Here's how the part is built. I have some questions about the finished solid (model axes, mm). Coordinates: 2 decimals unless noted, no trailing zeros. Order: outer loops, then holes, each group sorted by start corner. A loop starts at its lowest first (then second) coordinate and runs counter-clockwise, first axis right, second up.
```python
from build123d import *

# Parameters (mm, degrees)
SKETCH_1_R      = 12.5
SKETCH_1_R_2    = 4
SKETCH_1_R_3    = 1.5
SKETCH_1_R_4    = 1
SKETCH_1_R_5    = 0.5
EXTRUDE_1_DEPTH = 1


with BuildPart() as part:
    # Эскиз1 → Бобышка-Вытянуть1 (new body)
    with BuildSketch(Plane.XY):
        Circle(SKETCH_1_R)
        Circle(SKETCH_1_R_2, mode=Mode.SUBTRACT)
        with Locations((0, 9)):
            Circle(SKETCH_1_R_3, mode=Mode.SUBTRACT)
        with Locations((7.794228634, 4.5)):
            Circle(SKETCH_1_R_3, mode=Mode.SUBTRACT)
        with Locations((7.794228634, -4.5)):
            Circle(SKETCH_1_R_3, mode=Mode.SUBTRACT)
        with Locations((0, -9)):
            Circle(SKETCH_1_R_3, mode=Mode.SUBTRACT)
        with Locations((-7.794228634, -4.5)):
            Circle(SKETCH_1_R_3, mode=Mode.SUBTRACT)
        with Locations((-7.794228634, 4.5)):
            Circle(SKETCH_1_R_3, mode=Mode.SUBTRACT)
        with Locations((-5.5, 0)):
            Circle(SKETCH_1_R_4, mode=Mode.SUBTRACT)
        with Locations(Location((5.5, 0, 0), (0, 0, 180))):
            Circle(SKETCH_1_R_4, mode=Mode.SUBTRACT)
        with Locations((0, 5.5)):
            Circle(SKETCH_1_R_5, mode=Mode.SUBTRACT)
        with Locations((1.881110788, 5.168309414)):
            Circle(SKETCH_1_R_5, mode=Mode.SUBTRACT)
        with Locations((3.535331853, 4.213244437)):
            Circle(SKETCH_1_R_5, mode=Mode.SUBTRACT)
        with Locations((4.763139721, 2.75)):
            Circle(SKETCH_1_R_5, mode=Mode.SUBTRACT)
        with Locations((4.763139721, -2.75)):
            Circle(SKETCH_1_R_5, mode=Mode.SUBTRACT)
        with Locations((3.535331853, -4.213244437)):
            Circle(SKETCH_1_R_5, mode=Mode.SUBTRACT)
        with Locations((1.881110788, -5.168309414)):
            Circle(SKETCH_1_R_5, mode=Mode.SUBTRACT)
        with Locations((0, -5.5)):
            Circle(SKETCH_1_R_5, mode=Mode.SUBTRACT)
        with Locations((-1.881110788, -5.168309414)):
            Circle(SKETCH_1_R_5, mode=Mode.SUBTRACT)
        with Locations((-3.535331853, -4.213244437)):
            Circle(SKETCH_1_R_5, mode=Mode.SUBTRACT)
        with Locations((-4.763139721, -2.75)):
            Circle(SKETCH_1_R_5, mode=Mode.SUBTRACT)
        with Locations((-4.763139721, 2.75)):
            Circle(SKETCH_1_R_5, mode=Mode.SUBTRACT)
        with Locations((-3.535331853, 4.213244437)):
            Circle(SKETCH_1_R_5, mode=Mode.SUBTRACT)
        with Locations((-1.881110788, 5.168309414)):
            Circle(SKETCH_1_R_5, mode=Mode.SUBTRACT)
    extrude(amount=EXTRUDE_1_DEPTH)


solid = part.part
```
Q1. I need wall thicknesses on L1, parallel to Y at x = 2.25, z = 0.5; L2, parallel to X at y = -2.5, z = 0.4; L3, parallel to Y at x = 1, z = 0.55. Which ranges of each line are inside material? Lowest first, please.
Q2. Will this pin go through, and if not, where does the flat tip stop? pin 1 (1.8 mm diameter, centred on x = -7.79, y = -4.5, fed in from +Z).
Q3. If we section it at B-B on x = 0: Write out the boundary of the cut face in (y, z).
Q4. If we section it at A-A on y = 0: Write out the boundary of the cut face in (x, z).
Q5. If we section it at D-D on y = 9: Write out the boundary of the cut face in (x, z).
Q6. We'd pull the mould along Y, two halves only. Please class faces 1 (the cylindrical face through (11.923, 3.755, 0.493)), 2 (the cylindrical face through (-6.363, 4.951, 0.493)), 3 (the cylindrical face through (4.395, 3.088, 0.493)), 4 (the flat face through (-3, 3, 1)): pulls with the +Y half, pulls with the -Y half, needs draft (parallel to the pull), parting line crosses it, or undercut.
Q7. If we section it at C-C on z = 0.75: Give the number of separate pieces and of enclosed holes in the cut face, then the cut area to 3 significant figures.
Reply:
1. L1: y = -12.3 to -5.51, -4.83 to -3.31, 3.31 to 4.83, 5.51 to 12.3
1. L2: x = -12.25 to -5.2, -4.33 to -3.12, 3.12 to 4.33, 5.2 to 12.25
1. L3: y = -12.46 to -10.12, -7.88 to -3.87, 3.87 to 7.88, 10.12 to 12.46
2. pin 1: passes through
3. outline: (-12.5, 0) - (-10.5, 0) - (-10.5, 1) - (-12.5, 1) - close; (-7.5, 0) - (-6, 0) - (-6, 1) - (-7.5, 1) - close; (-5, 0) - (-4, 0) - (-4, 1) - (-5, 1) - close; (4, 0) - (5, 0) - (5, 1) - (4, 1) - close; (6, 0) - (7.5, 0) - (7.5, 1) - (6, 1) - close; (10.5, 0) - (12.5, 0) - (12.5, 1) - (10.5, 1) - close
4. outline: (-12.5, 0) - (-6.5, 0) - (-6.5, 1) - (-12.5, 1) - close; (-4.5, 0) - (-4, 0) - (-4, 1) - (-4.5, 1) - close; (4, 0) - (4.5, 0) - (4.5, 1) - (4, 1) - close; (6.5, 0) - (12.5, 0) - (12.5, 1) - (6.5, 1) - close
5. outline: (-8.67, 0) - (-1.5, 0) - (-1.5, 1) - (-8.67, 1) - close; (1.5, 0) - (8.67, 0) - (8.67, 1) - (1.5, 1) - close
6. face 1: parting line crosses it
6. face 2: undercut
6. face 3: undercut
6. face 4: needs draft
7. separate pieces: 1
7. enclosed holes: 23
7. area: 381 mm2
